Design review of the part built by this model. Coordinates are the model's own, in mm. A direction names the side the tool comes from. Give positions to 0.01 mm unless a question says otherwise; leave off trailing zeros. Write each loop counter-clockwise with the first axis right and the second up, starting at its lowest first coordinate (ties: lowest second). Pieces come first, ordered by that corner, then holes.
```python
from build123d import *

# Parameters (mm, degrees)
BOSS_EXTRUDE1_DEPTH = 10.16
SKETCH2_R           = 2.413
CUT_EXTRUDE1_DEPTH  = 7.4393


with BuildPart() as part:
    # Sketch1 → Boss-Extrude1 (new body)
    with BuildSketch(Plane(origin=(0, 0, 0), x_dir=(1, 0, 0), z_dir=(0, 1, 0))):
        with BuildLine():
            Line((-4.3434, -5.2744), (-6.474794456, -5.2744))
            ThreePointArc((-6.474794456, -5.2744), (-6.988471476, -4.931171988), (-6.867945826, -4.32524863))
            Line((-6.867945826, -4.32524863), (-3.537902285, -0.995205089))
            ThreePointArc((-3.537902285, -0.995205089), (-2.657092893, -0.406667069), (-1.618107374, -0.2))
            Line((-1.618107374, -0.2), (1.618107374, -0.2))
            ThreePointArc((1.618107374, -0.2), (2.657092893, -0.406667069), (3.537902285, -0.995205089))
            Line((3.537902285, -0.995205089), (6.867945826, -4.32524863))
            ThreePointArc((6.867945826, -4.32524863), (6.988471476, -4.931171988), (6.474794456, -5.2744))
            Line((6.474794456, -5.2744), (4.343399971, -5.2744))
            ThreePointArc((4.343399971, -5.2744), (3.309975564, -5.66416341), (2.791332959, -6.6393))
            Line((2.791332959, -6.6393), (-2.791332988, -6.6393))
            ThreePointArc((-2.791332988, -6.6393), (-3.309975593, -5.66416341), (-4.3434, -5.2744))
        make_face()
    extrude(amount=BOSS_EXTRUDE1_DEPTH)

    # Sketch2 → Cut-Extrude1 (cut, through all)
    with BuildSketch(Plane.XY.offset(6.6393)):
        with Locations((-1.4e-08, 5.08)):
            Circle(SKETCH2_R)
    extrude(amount=-CUT_EXTRUDE1_DEPTH, mode=Mode.SUBTRACT)


solid = part.part
```
(1) Consider section B-B, the plane y = 6.25. Give the boundary of the cut face in (x, z) (3 decimals).
Resolved:
outline: (-6.868, 4.325) - (-3.538, 0.995) arc R2.715 ccw to (-2.11, 0.245) - (-2.11, 6.639) - (-2.791, 6.639) arc R1.565 cw to (-4.343, 5.274) - (-6.475, 5.274) arc R0.556 ccw to start; (2.11, 0.245) arc R2.715 ccw to (3.538, 0.995) - (6.868, 4.325) arc R0.556 ccw to (6.475, 5.274) - (4.343, 5.274) arc R1.565 cw to (2.791, 6.639) - (2.11, 6.639) - close
(2) Consider section A-A, the plane x = 1. Give the boundary of the cut face in (y, z).
Resolved:
outline: (0, 0.2) - (2.88, 0.2) - (2.88, 6.64) - (0, 6.64) - close; (7.28, 0.2) - (10.16, 0.2) - (10.16, 6.64) - (7.28, 6.64) - close
(3) To check wall thickness, follow L1, parallel to X at y = 5.08, z = 4.75; L2, parallel to Y at x = 0, z = 5; L3, parallel to X at y = 3.5, z = 2.5. State the ranges of each line that lie inside material, in increasing order.
Resolved:
L1: x = -7.03 to -2.41, 2.41 to 7.03
L2: y = 0 to 2.67, 7.49 to 10.16
L3: x = -5.04 to -1.82, 1.82 to 5.04
(4) Consider section D-D, the plane z = 0.75. Give the boundary of the cut face in (x, y), then the cut area to 3 significant figures.
Resolved:
outline: (-3.26, 0) - (3.26, 0) - (3.26, 10.16) - (-3.26, 10.16) - close; hole circle Ø4.83 at (0, 5.08)
area: 47.9 mm2
(5) Consider section C-C, the plane y = 8. Give the boundary of the cut face in (x, z) (3 decimals).
Resolved:
outline: (-6.868, 4.325) - (-3.538, 0.995) arc R2.715 ccw to (-1.618, 0.2) - (1.618, 0.2) arc R2.715 ccw to (3.538, 0.995) - (6.868, 4.325) arc R0.556 ccw to (6.475, 5.274) - (4.343, 5.274) arc R1.565 cw to (2.791, 6.639) - (-2.791, 6.639) arc R1.565 cw to (-4.343, 5.274) - (-6.475, 5.274) arc R0.556 ccw to start
(6) Clearance check with flat-ended pins moving along their axes: P1, Ø1, axis at x = 2.5, y = 5.5, coming from the -Z side; P2, Ø2, axis at x = -5.5, y = 2.5, coming from the +Z side; P3, Ø1, axis at y = 5, z = 1.5, coming from the -X side. State where each tip first meets the part, or that it passes through.
Resolved:
P1: stops at z = 0.28
P2: stops at z = 5.27
P3: stops at x = -4.54
(7) Tool access review of faces 5 (the face through (0, 10.16, 3)), 6 (the face through (-5, 5, 5.274)), 7 (the face through (5, 5, 5.274)): name each direction out of +Z, -Z, +X, -X, +Y, -Y from which nothing blocks a thin tool from reaching the whole face with its end or side.
Resolved:
face 5: +Z, -Z, +X, -X, +Y
face 6: +Z, -X, +Y, -Y
face 7: +Z, +X, +Y, -Y
(8) Mouldability with a two-part tool opening along X and no side actions: class faces 1 (the face through (-7, 5, 4.9)), 2 (the face through (-0.523, 2.724, 3.465)), 3 (the face through (0, 9, 0.2)), 4 (the face through (2.64, 5.01, 0.4)) as pulls with the +X half, pulls with the -X half, needs draft (parallel to the pull), parting line crosses it, or undercut.
Resolved:
face 1: pulls with the -X half
face 2: undercut
face 3: needs draft
face 4: pulls with the +X half
